```python
from build123d import *

# Parameters (mm, degrees)
SKETCH1_W           = 47.974978614
SKETCH1_H           = 55.2
BOSS_EXTRUDE1_DEPTH = 3
SKETCH3_R           = 18.5
CUT_EXTRUDE2_DEPTH  = 8
SKETCH7_W           = 0.709516438
SKETCH7_H           = 55.2
SKETCH7_W_2         = 1.2
BOSS_EXTRUDE2_DEPTH = 2
SKETCH8_W           = 46.065462176
SKETCH8_H           = 0.744802826
SKETCH8_H_2         = 1.099561045
BOSS_EXTRUDE3_DEPTH = 2
SKETCH9_R           = 2
CUT_EXTRUDE4_DEPTH  = 2.5


with BuildPart() as part:
    # Sketch1 → Boss-Extrude1 (new body)
    with BuildSketch(Plane(origin=(0, 0, 0), x_dir=(1, 0, 0), z_dir=(0, 1, 0))):
        with Locations((-0.987489307, 0)):
            Rectangle(SKETCH1_W, SKETCH1_H)
    extrude(amount=BOSS_EXTRUDE1_DEPTH)

    # Sketch3 → Cut-Extrude2 (cut)
    with BuildSketch(Plane(origin=(0, 3, 0), x_dir=(1, 0, 0), z_dir=(0, 1, 0))):
        with Locations(Location((0, 0, 0), (0, 0, 270))):
            Circle(SKETCH3_R)
    extrude(amount=-CUT_EXTRUDE2_DEPTH, mode=Mode.SUBTRACT)

    # Sketch7 → Boss-Extrude2 (add)
    with BuildSketch(Plane.XZ):
        with Locations((-24.620220395, 0)):
            Rectangle(SKETCH7_W, SKETCH7_H)
        with Locations((22.4, 0)):
            Rectangle(SKETCH7_W_2, SKETCH7_H)
    extrude(amount=BOSS_EXTRUDE2_DEPTH)

    # Sketch8 → Boss-Extrude3 (add)
    with BuildSketch(Plane.XZ):
        with Locations((-1.232731088, 27.227598587)):
            Rectangle(SKETCH8_W, SKETCH8_H)
        with Locations((-1.232731088, -27.050219478)):
            Rectangle(SKETCH8_W, SKETCH8_H_2)
    extrude(amount=BOSS_EXTRUDE3_DEPTH)

    # Sketch9 → Cut-Extrude4 (cut)
    with BuildSketch(Plane.XZ):
        with Locations(Location((-19.324035892, 18.962761771, 0), (0, 0, 270))):
            Circle(SKETCH9_R)
        with Locations(Location((18.115964108, 18.962761771, 0), (0, 0, 270))):
            Circle(SKETCH9_R)
        with Locations(Location((-19.324035892, -18.477238229, 0), (0, 0, 270))):
            Circle(SKETCH9_R)
        with Locations(Location((18.115964108, -18.477238229, 0), (0, 0, 270))):
            Circle(SKETCH9_R)
    extrude(amount=-CUT_EXTRUDE4_DEPTH, mode=Mode.SUBTRACT)


solid = part.part
```
Can you work these out from the model? Positions are in its coordinate system, mm. A direction names the side the tool comes from. Coordinates: 2 decimals unless noted, no trailing zeros. Loops run counter-clockwise (first coordinate to the right, second up) from the corner with the lowest first, then second, coordinate; pieces in that order, holes last.
1) Imagine slicing it at D-D on y = 1.3. List the corners of the cut face in (x, z) for me, plus the area to 3 significant figures.
2) Thinking about a two-plate mould opening in Z: for faces 1 (the flat face through (-24.975, 1, 0)), 2 (the flat face through (-1, 1, -27.6)), 3 (the cylindrical face through (19.468, 1.232, 20.437)), which applies, pulls with the +Z half, pulls with the -Z half, needs draft (parallel to the pull), parting line crosses it, or undercut?
3) I need wall thicknesses on probe 1 along Z at (x, y) = (-20, 2.25); probe 2 along X at (y, z) = (2.15, 20); probe 3 along X at (y, z) = (-0.35, 21.5). Which ranges of each line are inside material? Lowest first, please.
4) Imagine slicing it at B-B on x = 0. List the corners of the cut face in (y, z) for me.
5) Imagine slicing it at C-C on z = 23.5. List the corners of the cut face in (x, y) for me.
6) For pin 1 (14 mm diameter, centred on x = 9, z = -2.5, fed in from -Y); pin 2 (5 mm diameter, centred on x = -19.32, z = -18.48, fed in from -Y); pin 3 (1.2 mm diameter, centred on x = 18.5, z = 18.5, fed in from -Y), each with a flat end and sliding along its axis, tell me the tip position at first contact or that it passes through.
7) Which directions (+Z, -Z, +X, -X, +Y, -Y) give clear straight access to the entire face, cutting with the end or side of a thin tool? Please do faces 4 (the cylindrical face through (20.1, 1.23, -18.22)), 5 (the flat face through (22, -2, 0)).
8) Imagine slicing it at A-A on z = 0. List the corners of the cut face in (x, y) for me.
Completed:
1. outline: (-24.97, -27.6) - (23, -27.6) - (23, 27.6) - (-24.97, 27.6) - close; hole circle Ø4 at (-19.32, -18.48); hole circle Ø4 at (-19.32, 18.96); hole circle Ø37 at (0, 0); hole circle Ø4 at (18.12, -18.48); hole circle Ø4 at (18.12, 18.96)
1. area: 1,520 mm2
2. face 1: needs draft
2. face 2: pulls with the -Z half
2. face 3: undercut
3. probe 1: z = -27.6 to -20.36, -16.59 to 17.08, 20.85 to 27.6
3. probe 2: x = -24.97 to -21.03, -17.61 to 16.41, 19.83 to 23
3. probe 3: x = -24.97 to -24.27, 21.8 to 23
4. outline: (-2, -27.6) - (3, -27.6) - (3, -18.5) - (0, -18.5) - (0, -26.5) - (-2, -26.5) - close; (-2, 26.86) - (0, 26.86) - (0, 18.5) - (3, 18.5) - (3, 27.6) - (-2, 27.6) - close
5. outline: (-24.97, -2) - (-24.27, -2) - (-24.27, 0) - (21.8, 0) - (21.8, -2) - (23, -2) - (23, 3) - (-24.97, 3) - close
6. pin 1: passes through
6. pin 2: stops at y = 0
6. pin 3: stops at y = 2.5
7. face 4: -Y
7. face 5: +Z, -Z, +X, -X, -Y
8. outline: (-24.97, -2) - (-24.27, -2) - (-24.27, 0) - (-18.5, 0) - (-18.5, 3) - (-24.97, 3) - close; (18.5, 0) - (21.8, 0) - (21.8, -2) - (23, -2) - (23, 3) - (18.5, 3) - close
